Here's how the part is built. I have some questions about the finished solid (model axes, mm). Face numbers are marked on the shaded views. Round coordinates to 2 decimals unless told otherwise and drop trailing zeros. Write each loop counter-clockwise with the first axis right and the second up, starting at its lowest first coordinate (ties: lowest second). Pieces come first, ordered by that corner, then holes. Notation, with made-up numbers: M 80.25,52 L 99.25,52 A25 cw 99.25,85 Z; hole C 60.5,-21 d3. An arc over 180 degrees is marked long. Write item = value, one per line. Start each with the question number.
(1) I need wall thicknesses on line 1 along X through (y, z) = (77, 0); line 2 along Y through (x, z) = (12, 5); line 3 along Y through (x, z) = (-12, 6). Which ranges of each line are inside material? Lowest first, please.
(2) Will these pins go through, and if not, where does the flat tip stop? pin 1 Ø5 at (y, z) = (30.5, 19.5) entering from -X; pin 2 Ø12 at (y, z) = (105.5, 19) entering from -X; pin 3 Ø4 at (y, z) = (40.5, -6) entering from -X.
(3) If we mould it in two halves opening along Z, with no side actions, what happens to the marked faces 1, 2 and 3? For each: released by +Z, released by -Z, zero draft, split by the parting line, or undercut.
(4) I want a section at A-A (y = 60.5). List the corners of the cut face in (x, z) for me.
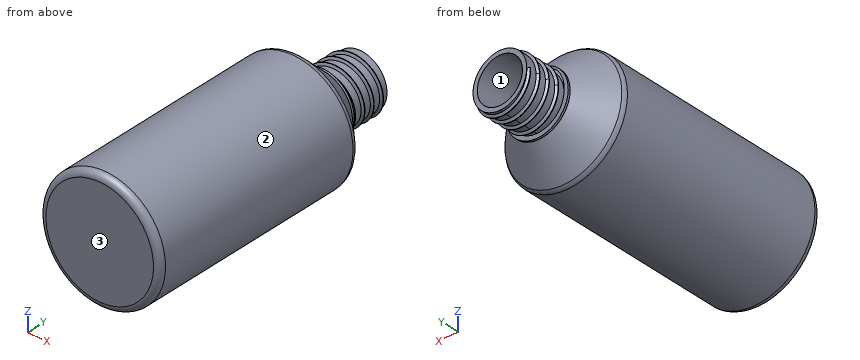
```python
from build123d import *

# Parameters (mm, degrees)
RADYUS1_R  = 3
DI_1_PITCH = 5


# Read off the part's stored shape, not the designer's step: İç Boşaltma1
with BuildPart() as part:
    # Çizim1 → Döndür1 (revolve)
    with BuildSketch(Plane.XY, mode=Mode.PRIVATE) as d_nd_r1_sk:
        Polygon((0, 0), (-28, 0), (-28, 105), (-14.5, 119), (-14.5, 120), (-12.5, 120), (-12.5, 140), (0, 140), align=None)
    revolve(d_nd_r1_sk.sketch.rotate(Axis((0, 0, 0), (0, 1, 0)), 270), axis=Axis((0, 0, 0), (0, 1, 0)))

    # Radyus1
    radyus1_edges = [part.edges().sort_by_distance(p)[0] for p in [
        (0, 105, 28),
        (0, 0, 28),
    ]]
    fillet(radyus1_edges, radius=RADYUS1_R)

    # İç Boşaltma1 outline → İç Boşaltma1 (revolve, cut)
    with BuildSketch(Plane.XY):
        with BuildLine():
            Line((0, 140), (0, 2))
            Line((0, 2), (25, 2))
            ThreePointArc((25, 2), (25.707106781, 2.292893219), (26, 3))
            Line((26, 3), (26, 103.789188814))
            ThreePointArc((26, 103.789188814), (25.927319873, 104.163458572), (25.719844295, 104.483324384))
            Line((25.719844295, 104.483324384), (12.685907094, 118))
            Line((12.685907094, 118), (10.5, 118))
            Line((10.5, 118), (10.5, 140))
            Line((10.5, 140), (0, 140))
        make_face()
    revolve(axis=Axis((0, 0, 0), (0, 1, 0)), mode=Mode.SUBTRACT)

    # Diş1: the profile of Diş Profili1 profile screwed along a right-hand helix of 4 turns, 12 arcs to a turn; built about Z, then put on its axis
    di_1_z = Axis((0, 0, 0), (0, 0, 1))
    di_1_corners = [(12.4997, 0, -0.000173205), (13.58253175, 0, 0.624999997), (13.58253175, 0, 0.874999997), (12.4997, 0, 1.5001732)]
    with BuildLine(mode=Mode.PRIVATE) as di_1_profile:
        Line(di_1_corners[0], di_1_corners[1])
        Line(di_1_corners[1], di_1_corners[2])
        Line(di_1_corners[2], di_1_corners[3])
        Line(di_1_corners[3], di_1_corners[0])
    di_1_cap = Face(di_1_profile.wire())
    di_1_turn_angles = [0, 15, 30, 45, 60, 75, 90, 105, 120, 135, 150, 165, 180, 195, 210, 225, 240, 255, 270, 285, 300, 315, 330, 345, 360]
    di_1_turn_weights = [1, 0.9659258262890683, 1, 0.9659258262890683, 1, 0.9659258262890683, 1, 0.9659258262890683, 1, 0.9659258262890683, 1, 0.9659258262890683, 1, 0.9659258262890683, 1, 0.9659258262890683, 1, 0.9659258262890683, 1, 0.9659258262890683, 1, 0.9659258262890683, 1, 0.9659258262890683, 1]
    di_1_turn_rails = [Edge.make_bspline([Vector(p[0], p[1], 0).rotate(di_1_z, di_1_turn_angles[k]) / di_1_turn_weights[k] + Vector(0, 0, p[2] + DI_1_PITCH * di_1_turn_angles[k] / 360) for k in range(25)], [0, 0, 0, 1, 1, 2, 2, 3, 3, 4, 4, 5, 5, 6, 6, 7, 7, 8, 8, 9, 9, 10, 10, 11, 11, 12, 12, 12], 2, di_1_turn_weights) for p in di_1_corners]
    di_1_turn_sides = [Face.make_surface_from_curves(di_1_turn_rails[p[0]], di_1_turn_rails[p[1]]) for p in [(0, 1), (1, 2), (2, 3), (3, 0)]]
    di_1 = Plane(origin=(0, 140, 0), x_dir=(-1, 0, 0), z_dir=(0, -1, 0)) * Solid(Shell([*[p.moved(Location((0, 0, DI_1_PITCH * i))) for i in range(4) for p in di_1_turn_sides], di_1_cap, di_1_cap.rotate(di_1_z, 1440).moved(Location((0, 0, DI_1_PITCH * 1440 / 360)))]))
    add(di_1)


solid = part.part
```
Returned:
q1.line_1 = -28 to -26, 26 to 28
q1.line_2 = 0 to 2, 117.67 to 120, 120.97 to 121.9, 125.97 to 126.9, 130.97 to 131.9, 135.97 to 136.9
q1.line_3 = 0 to 2, 117.24 to 120, 124.4 to 124.84, 129.4 to 129.84, 134.4 to 134.84
q2.pin_1 = -22.25
q2.pin_2 = -24.69
q2.pin_3 = -27.71
q3.face_1 = undercut
q3.face_2 = split by the parting line
q3.face_3 = zero draft
q4.outline = C 0,0 d56; hole C 0,0 d52
